Part model, mm, in its own coordinate system. Give positions to 0.01 mm unless a question says otherwise; leave off trailing zeros. Write each loop counter-clockwise with the first axis right and the second up, starting at its lowest first coordinate (ties: lowest second). Pieces come first, ordered by that corner, then holes. Notation, with made-up numbers: M 49.25,34.25 L 108.25,34.25 A18 cw 108.25,55.25 Z; hole C 35,60 d11. An arc over 180 degrees is marked long. Write item = value, one per line. Start each with the question number.
from build123d import *

# Parameters (mm, degrees)
SKETCH1_W           = 105
SKETCH1_H           = 76
SKETCH1_W_2         = 85
SKETCH1_H_2         = 56
SKETCH1_R           = 2.5
BOSS_EXTRUDE1_DEPTH = 10


with BuildPart() as part:
    # Sketch1 → Boss-Extrude1 (new body)
    with BuildSketch(Plane.XY):
        Rectangle(SKETCH1_W, SKETCH1_H)
        Rectangle(SKETCH1_W_2, SKETCH1_H_2, mode=Mode.SUBTRACT)
        Rectangle(SKETCH1_W_2, SKETCH1_H_2)
        with Locations((-39, -24.5)):
            Circle(SKETCH1_R, mode=Mode.SUBTRACT)
        with Locations((19, -24.5)):
            Circle(SKETCH1_R, mode=Mode.SUBTRACT)
        with Locations((-39, 24.5)):
            Circle(SKETCH1_R, mode=Mode.SUBTRACT)
        with Locations((19, 24.5)):
            Circle(SKETCH1_R, mode=Mode.SUBTRACT)
    extrude(amount=BOSS_EXTRUDE1_DEPTH)


solid = part.part
Q1. Slice it at B-B (y = -24.5). Give the cut face in (x, z).
Q2. Probe line 1 along Y through (x, z) = (19, 4); line 2 along Y through (x, z) = (18, 6). List the from-to ranges inside material, lowest first.
Q3. Two-plate mould, pull along X, no slides. Class faces 1 (the face through (-52.5, -1, 5)), 2 (the face through (-1, 38, 5)), 3 (the face through (52.5, -1, 5)), 4 (the face through (17, 26, 5)): +X half, -X half, draft (parallel to the pull), parting line (faces both ways), or undercut.
Q4. Slice it at A-A (x = 19). Give the cut face in (y, z).
Working result:
q1.outline = M -52.5,0 L -41.5,0 L -41.5,10 L -52.5,10 Z; M -36.5,0 L 16.5,0 L 16.5,10 L -36.5,10 Z; M 21.5,0 L 52.5,0 L 52.5,10 L 21.5,10 Z
q2.line_1 = -38 to -27, -22 to 22, 27 to 38
q2.line_2 = -38 to -26.79, -22.21 to 22.21, 26.79 to 38
q3.face_1 = -X half
q3.face_2 = draft
q3.face_3 = +X half
q3.face_4 = undercut
q4.outline = M -38,0 L -27,0 L -27,10 L -38,10 Z; M -22,0 L 22,0 L 22,10 L -22,10 Z; M 27,0 L 38,0 L 38,10 L 27,10 Z
